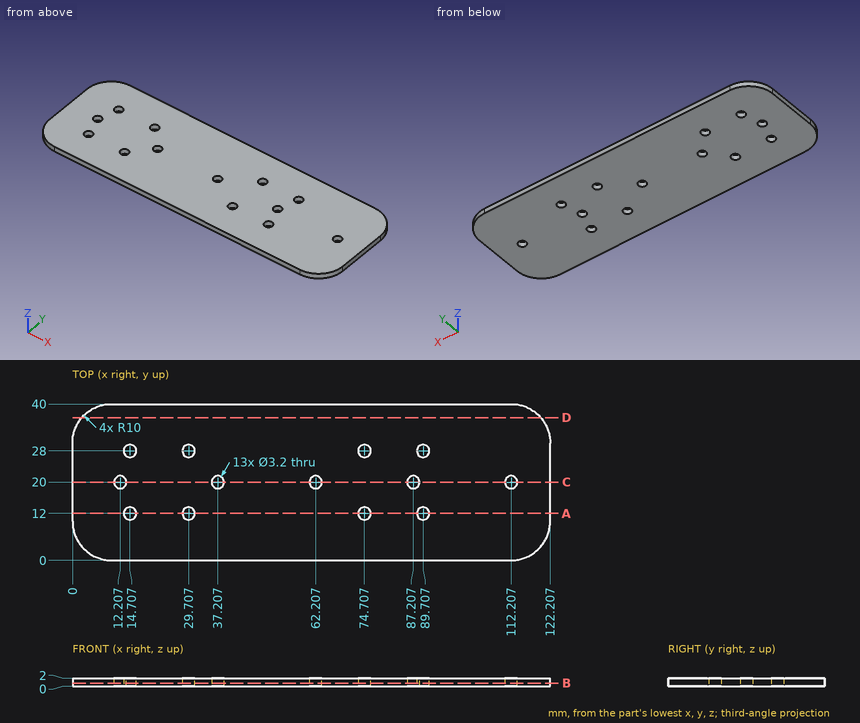
Input: dimensioned drawing with shaded views. Units: mm. Origin: part minimum x, y, z. Give positions to 0.01 mm unless a question says otherwise; leave off trailing zeros. Write each loop counter-clockwise with the first axis right and the second up, starting at its lowest first coordinate (ties: lowest second). Pieces come first, ordered by that corner, then holes. Notation, with made-up numbers: M 14.5,70 L 51.5,70 A21 cw 51.5,93 Z; hole C 76,40 d10. An arc over 180 degrees is marked long. Write item = value, one per line. Start each with the question number.
1) Cut plane A-A on y = 12. Return the cut outline in (x, z).
2) Cut plane B-B on z = 0.8. Count the separate pieces of the cut face and the enclosed holes in it, then the cut area to 3 significant figures.
3) First-contact query: pin 1 Ø3 at (x, y) = (74.71, 12) entering from -Z. Flat tip, straight axial feed; report the tip coordinate or a pass-through.
4) Cut plane D-D on y = 36.5. Return the cut outline in (x, z).
5) Material intervals for line 1 along Y through (x, z) = (74, 0.45) (1 decimal); line 2 along X through (y, z) = (32, 0.2) (1 decimal); line 3 along Y through (x, z) = (7, 0.1), sorted ascending. Write a range as [from, to].
6) Cut plane C-C on y = 20. Return the cut outline in (x, z).
Solved:
q1.outline = M 0,0 L 13.11,0 L 13.11,2 L 0,2 Z; M 16.31,0 L 28.11,0 L 28.11,2 L 16.31,2 Z; M 31.31,0 L 73.11,0 L 73.11,2 L 31.31,2 Z; M 76.31,0 L 88.11,0 L 88.11,2 L 76.31,2 Z; M 91.31,0 L 122.21,0 L 122.21,2 L 91.31,2 Z
q2.separate_pieces = 1
q2.enclosed_holes = 13
q2.area = 4,700 mm2
q3.pin_1 = through
q4.outline = M 2.4,0 L 119.81,0 L 119.81,2 L 2.4,2 Z
q5.line_1 = [0, 10.6], [13.4, 26.6], [29.4, 40]
q5.line_2 = [0.2, 122]
q5.line_3 = [0.46, 39.54]
q6.outline = M 0,0 L 10.61,0 L 10.61,2 L 0,2 Z; M 13.81,0 L 35.61,0 L 35.61,2 L 13.81,2 Z; M 38.81,0 L 60.61,0 L 60.61,2 L 38.81,2 Z; M 63.81,0 L 85.61,0 L 85.61,2 L 63.81,2 Z; M 88.81,0 L 110.61,0 L 110.61,2 L 88.81,2 Z; M 113.81,0 L 122.21,0 L 122.21,2 L 113.81,2 Z
